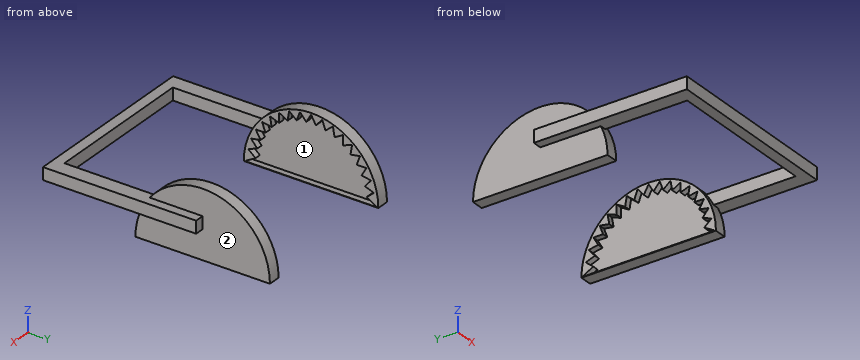
```python
from build123d import *

# Parameters (mm, degrees)
F0_W      = 40
F0_H      = 60
F1_DEPTH  = 20
F2_W      = 26
F2_H      = 58
F3_DEPTH  = 10
F5_DEPTH  = 5
F14_DEPTH = 4
F15_DEPTH = 2
F16_DEPTH = 4
F17_DEPTH = 2
F20_DEPTH = 2


with BuildPart() as f1:
    # F0 (on Top) → F1 (new body)
    with BuildSketch(Plane.XY):
        Rectangle(F0_W, F0_H)
    extrude(amount=F1_DEPTH)

    # F2 (on face) → F3 (cut)
    with BuildSketch(Plane.XY.offset(20)):
        with Locations((0, -1)):
            Rectangle(F2_W, F2_H)
    extrude(amount=-F3_DEPTH, mode=Mode.SUBTRACT)

    # F4 (on face) → F5 (join)
    with BuildSketch(Plane.YZ.offset(20)):
        Polygon((10, 17.3205080757), (7.368124542, 15.8009940716), (6.8404028665, 18.7938524157), (4.5123723483, 16.8404028665), (3.4729635533, 19.6961550602), (1.5195140041, 17.368124542), (0, 20), (-1.5195140041, 17.368124542), (-3.4729635533, 19.6961550602), (-4.5123723483, 16.8404028665), (-6.8404028665, 18.7938524157), (-7.368124542, 15.8009940716), (-10, 17.3205080757), (-10, 14.2814800674), (-12.8557521937, 15.3208888624), (-12.3280305182, 12.3280305182), (-15.3208888624, 12.8557521937), (-14.2814800674, 10), (-17.3205080757, 10), (-15.8009940716, 7.368124542), (-18.7938524157, 6.8404028665), (-16.8404028665, 4.5123723483), (-19.6961550602, 3.4729635533), (-17.368124542, 1.5195140041), (-20, 0), (20, 0), (17.368124542, 1.5195140041), (19.6961550602, 3.4729635533), (16.8404028665, 4.5123723483), (18.7938524157, 6.8404028665), (15.8009940716, 7.368124542), (17.3205080757, 10), (14.2814800674, 10), (15.3208888624, 12.8557521937), (12.3280305182, 12.3280305182), (12.8557521937, 15.3208888624), (10, 14.2814800674), align=None)
    extrude(amount=F5_DEPTH)

    # F6: F1 across plane


with BuildPart() as f1_1:
    add(f1.part)
    add(f1.part.mirror(Plane.YZ))


with BuildPart() as f14:
    # F12 (on offset) → F14 (new body)
    with BuildSketch(Plane.YZ.offset(-23)):
        with BuildLine():
            Line((-21.9604505755, -11.5237375721), (21.9604505755, -11.5237375721))
            ThreePointArc((21.9604505755, -11.5237375721), (0, 10.4367130033), (-21.9604505755, -11.5237375721))
        make_face()
    extrude(amount=-F14_DEPTH)


with BuildPart() as f15_tool:
    # F10 (on offset) → F15 (new body)
    with BuildSketch(Plane.YZ.offset(-23)):
        Polygon((13.4108637106, 4.9916980332), (10.4318001067, 3.9074075554), (10.4318001067, 7.0776608255), (7.6862802384, 5.4925341904), (7.1357715353, 8.6146241898), (4.7072166344, 6.5768246682), (3.6229261566, 9.5558882722), (1.585126635, 7.1273333713), (0, 9.8728532397), (-1.585126635, 7.1273333713), (-3.6229261566, 9.5558882722), (-4.7072166344, 6.5768246682), (-7.1357715353, 8.6146241898), (-7.6862802384, 5.4925341904), (-10.4318001067, 7.0776608255), (-10.4318001067, 3.9074075554), (-13.4108637106, 4.9916980332), (-12.8603550075, 1.8696080338), (-15.9824450069, 2.4201167369), (-14.8981545291, -0.558946867), (-18.0684077992, -0.558946867), (-16.4832811642, -3.3044667354), (-19.6053711636, -3.8549754385), (-17.567571642, -6.2835303393), (-20.5466352459, -7.3678208171), (-18.1180803451, -9.4056203387), (-21.6114999369, -11.4225470804), (21.6114999369, -11.4225470804), (18.1180803451, -9.4056203387), (20.5466352459, -7.3678208171), (17.567571642, -6.2835303393), (19.6053711636, -3.8549754385), (16.4832811642, -3.3044667354), (18.0684077992, -0.558946867), (14.8981545291, -0.558946867), (15.9824450069, 2.4201167369), (12.8603550075, 1.8696080338), align=None)
    extrude(amount=-F15_DEPTH)


with BuildPart() as f1_2:
    add(f1_1.part)

    # F15: cut by f15_tool
    add(f15_tool.part, mode=Mode.SUBTRACT)


with BuildPart() as f14_1:
    add(f14.part)

    # F15: cut by f15_tool
    add(f15_tool.part, mode=Mode.SUBTRACT)



with BuildPart() as f16:
    # F13 (on offset) → F16 (new body)
    with BuildSketch(Plane.YZ.offset(23)):
        with BuildLine():
            Line((-21.9604505755, -11.5237375721), (21.9604505755, -11.5237375721))
            ThreePointArc((21.9604505755, -11.5237375721), (0, 10.4367130033), (-21.9604505755, -11.5237375721))
        make_face()
    extrude(amount=F16_DEPTH)


with BuildPart() as f17_tool:
    # F11 (on offset) → F17 (new body)
    with BuildSketch(Plane.YZ.offset(23)):
        Polygon((13.4108637106, 5.0649986808), (10.4318001067, 3.980708203), (10.4318001067, 7.1509614731), (7.6862802384, 5.565834838), (7.1357715353, 8.6879248374), (4.7072166344, 6.6501253158), (3.6229261566, 9.6291889197), (1.585126635, 7.2006340189), (0, 9.9461538872), (-1.585126635, 7.2006340189), (-3.6229261566, 9.6291889197), (-4.7072166344, 6.6501253158), (-7.1357715353, 8.6879248374), (-7.6862802384, 5.565834838), (-10.4318001067, 7.1509614731), (-10.4318001067, 3.980708203), (-13.4108637106, 5.0649986808), (-12.8603550075, 1.9429086814), (-15.9824450069, 2.4934173845), (-14.8981545291, -0.4856462195), (-18.0684077992, -0.4856462195), (-16.4832811642, -3.2311660878), (-19.6053711636, -3.7816747909), (-17.567571642, -6.2102296917), (-20.5466352459, -7.2945201695), (-18.1180803451, -9.3323196911), (-21.6114999369, -11.3492464328), (21.6114999369, -11.3492464328), (18.1180803451, -9.3323196911), (20.5466352459, -7.2945201695), (17.567571642, -6.2102296917), (19.6053711636, -3.7816747909), (16.4832811642, -3.2311660878), (18.0684077992, -0.4856462195), (14.8981545291, -0.4856462195), (15.9824450069, 2.4934173845), (12.8603550075, 1.9429086814), align=None)
    extrude(amount=F17_DEPTH)


with BuildPart() as f1_3:
    add(f1_2.part)

    # F17: cut by f17_tool
    add(f17_tool.part, mode=Mode.SUBTRACT)


with BuildPart() as f16_1:
    add(f16.part)

    # F17: cut by f17_tool
    add(f17_tool.part, mode=Mode.SUBTRACT)


with BuildPart() as f14_2:
    add(f14_1.part)

    add(f16_1.part)  # F20 merges F16
    # F19 (on Top) → F20 (join, symmetric)
    with BuildSketch(Plane.XY):
        Polygon((-25, 0), (-30, 0), (-30, -50), (30, -50), (30, 0), (25, 0), (25, -46.5494953096), (-25, -46.5494953096), align=None)
    extrude(amount=F20_DEPTH, both=True)


solid = f14_2.part
```
The listing builds one solid part. Answer for the finished solid, in the listing's coordinates (mm). Face numbers are marked on the shaded views. Round coordinates to 2 decimals unless told otherwise and drop trailing zeros. Loops run counter-clockwise (first coordinate to the right, second up) from the corner with the lowest first, then second, coordinate; pieces in that order, holes last.
1) A cutting plane is placed at A-A on y = -45. Determine the outline of the cut face in (x, z).
Outcome:
outline: (-30, -2) - (-25, -2) - (-25, 2) - (-30, 2) - close; (25, -2) - (30, -2) - (30, 2) - (25, 2) - close
2) Given P1, Ø6.5, axis at y = -2.5, z = -5.5, coming from the -X side; P2, Ø2.5, axis at x = -28, z = 0, coming from the +Y side; P3, Ø5, axis at x = 0.5, z = -4, coming from the -Y side; P4, Ø2, axis at x = -23.5, z = 5, coming from the -Y side, each flat-ended and moving along its own axis, determine where each tip first touches the part or whether it passes through.
Outcome:
P1: stops at x = -27
P2: stops at y = 19.14
P3: stops at y = -50
P4: stops at y = -15.53
3) Consider line 1 (X direction, y = 5.5, z = -3.5); line 2 (X direction, y = -34, z = 0.25); line 3 (Y direction, x = 8, z = 1.5). Determine where each line is inside the solid, lowest interval first.
Outcome:
line 1: x = -27 to -25, 25 to 27
line 2: x = -30 to -25, 25 to 30
line 3: y = -50 to -46.55
4) A cutting plane is placed at B-B on x = -20.5. Determine the outline of the cut face in (y, z).
Outcome:
outline: (-50, -2) - (-46.55, -2) - (-46.55, 2) - (-50, 2) - close
5) For a pull along Z with two mould halves and no side action, classify the marked faces 1 and 2 as released by +Z, released by -Z, zero draft, split by the parting line, or undercut.
Outcome:
face 1: undercut
face 2: zero draft
